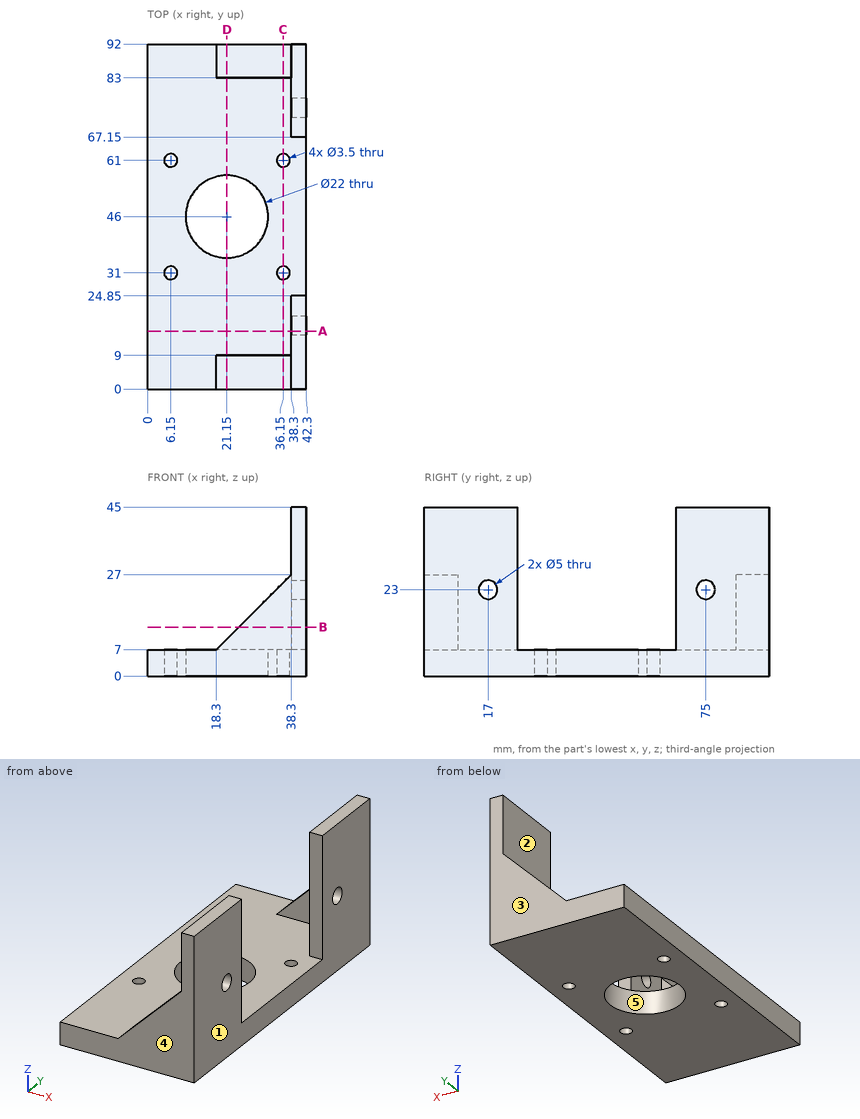
The drawing under review shows one solid part. Ordinate dimensions are in mm from its lowest x, y, z. A direction names the side the tool comes from. Coordinates: 2 decimals unless noted, no trailing zeros. Write each loop counter-clockwise with the first axis right and the second up, starting at its lowest first coordinate (ties: lowest second). Pieces come first, ordered by that corner, then holes. Notation, with made-up numbers: (-29.75, 46) -> (20.25, 46) arc R33 ccw to (20.25, 85) -> close; hole circle Ø3 at (76.25, 3.25). An arc over 180 degrees is marked (long way). One line per item, written item: value. Start each with the question number.
Q1. Add section B-B, the plane z = 13. Give the boundary of the cut face in (x, y), then the cut area to 3 significant figures.
Q2. Add section C-C, the plane x = 36.15. Give the boundary of the cut face in (y, z).
Q3. The part is to be moulded in two halves that separate along Y. For the marked faces 3, 4 and 5, say which applies: +Y half, -Y half, draft (parallel to the pull), parting line (faces both ways), or undercut.
Q4. Clearance check with flat-ended pins moving along their axes: P1, Ø4.5, axis at y = 75, z = 23, coming from the +X side; P2, Ø2, axis at x = 9.5, y = 42.5, coming from the +Z side; P3, Ø8, axis at y = 17, z = 23, coming from the -X side; P4, Ø20, axis at y = 83.5, z = 35, coming from the -X side. State where each tip first meets the part, or that it passes through.
Q5. For the marked faces 1 and 2, list the 3-axis set-ups (+Z, -Z, +X, -X, +Y, -Y) from which the entire face can be reached by the end or side of a thin tool; tool diameter is ignored.
Q6. Add section A-A, the plane y = 15.5. Give the boundary of the cut face in (x, z).
Q7. To check wall thickness, follow probe 1 along Y at (x, z) = (6.15, 5); probe 2 along Z at (x, y) = (39.6, 75); probe 3 along Y at (x, z) = (21.15, 5). State the ranges of each line that lie inside material, in increasing order.
Q8. Add section D-D, the plane x = 21.15. Give the boundary of the cut face in (y, z), then the cut area to 3 significant figures.
Response:
1. outline: (24.3, 0) -> (42.3, 0) -> (42.3, 24.85) -> (38.3, 24.85) -> (38.3, 9) -> (24.3, 9) -> close; (24.3, 83) -> (38.3, 83) -> (38.3, 67.15) -> (42.3, 67.15) -> (42.3, 92) -> (24.3, 92) -> close
1. area: 451 mm²
2. outline: (0, 0) -> (29.25, 0) -> (29.25, 7) -> (9, 7) -> (9, 24.85) -> (0, 24.85) -> close; (32.75, 0) -> (59.25, 0) -> (59.25, 7) -> (32.75, 7) -> close; (62.75, 0) -> (92, 0) -> (92, 24.85) -> (83, 24.85) -> (83, 7) -> (62.75, 7) -> close
3. face 3: +Y half
3. face 4: -Y half
3. face 5: undercut
4. P1: through
4. P2: z = 7
4. P3: x = 38.3
4. P4: x = 36.3
5. face 1: +Z, -Z, +X, +Y, -Y
5. face 2: +Z, -X
6. outline: (0, 0) -> (42.3, 0) -> (42.3, 21) -> (38.3, 21) -> (38.3, 7) -> (0, 7) -> close; (38.3, 25) -> (42.3, 25) -> (42.3, 45) -> (38.3, 45) -> close
7. probe 1: 0 to 29.25, 32.75 to 59.25, 62.75 to 92
7. probe 2: 0 to 20.5, 25.5 to 45
7. probe 3: 0 to 35, 57 to 92
8. outline: (0, 0) -> (35, 0) -> (35, 7) -> (9, 7) -> (9, 9.85) -> (0, 9.85) -> close; (57, 0) -> (92, 0) -> (92, 9.85) -> (83, 9.85) -> (83, 7) -> (57, 7) -> close
8. area: 541 mm²
